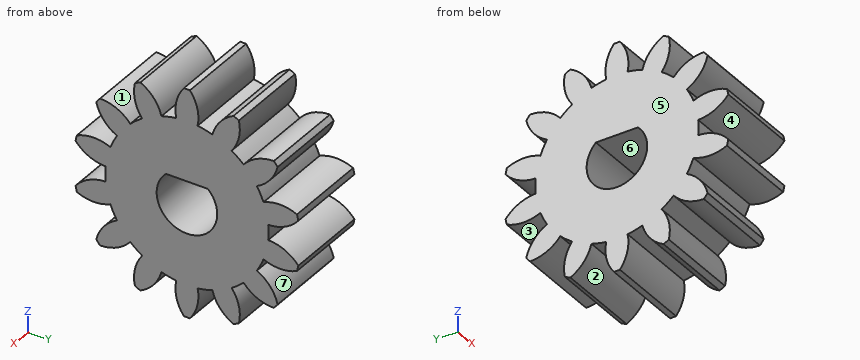
```python
from build123d import *

# Parameters (mm, degrees)
BASPROSKE_W         = 14
BASPROSKE_H         = 12
TOOTHCUT_DEPTH      = 23
TEETHCUTS_COUNT     = 14
TEETHCUTS_ANGLE     = 334.285714286
BORSKE_R            = 3
BORE_DEPTH          = 50.0000508
SKETCH2_R           = 16.086266861
CUT_EXTRUDE1_DEPTH  = 5
SKETCH3_R           = 3.2
CUT_EXTRUDE2_DEPTH  = 20.064015522
BOSS_EXTRUDE1_DEPTH = 9


with BuildPart() as part:
    # BasProSke → Base-Revolve (revolve)
    with BuildSketch(Plane(origin=(0, 0, 0), x_dir=(1, 0, 0), z_dir=(0, 1, 0)), mode=Mode.PRIVATE) as base_revolve_sk:
        with Locations((7, 6)):
            Rectangle(BASPROSKE_W, BASPROSKE_H)
    revolve(base_revolve_sk.sketch.rotate(Axis((-10, 0, 0), (1, 0, 0)), 180), axis=Axis((-10, 0, 0), (1, 0, 0)))

    # TooCutSke → ToothCut (cut, through all)
    with BuildSketch(Plane(origin=(0, 0, 0), x_dir=(0, 0, -1), z_dir=(1, 0, 0))):
        with BuildLine():
            ThreePointArc((0.804845511, 8.586361261), (0, 8.624), (-0.804845511, 8.586361261))
            ThreePointArc((-0.804845511, 8.586361261), (-1.237812142, 10.362618414), (-2.384428228, 11.78663426))
            ThreePointArc((-2.384428228, 11.78663426), (0, 12.0254), (2.384428228, 11.78663426))
            ThreePointArc((2.384428228, 11.78663426), (1.237812142, 10.362618414), (0.804845511, 8.586361261))
        make_face()
    toothcut = extrude(amount=TOOTHCUT_DEPTH, mode=Mode.SUBTRACT)

    # TeethCuts: ToothCut ×14 about axis
    teethcuts_axis = Axis((-10, 0, 0), (1, 0, 0))
    for i in range(1, TEETHCUTS_COUNT):
        add(toothcut.rotate(teethcuts_axis, i * TEETHCUTS_ANGLE / (TEETHCUTS_COUNT - 1)), mode=Mode.SUBTRACT)

    # BorSke → Bore (cut, symmetric)
    with BuildSketch(Plane(origin=(0, 0, 0), x_dir=(0, 0, -1), z_dir=(1, 0, 0))):
        with Locations(Location((0, 0, 0), (0, 0, 180))):
            Circle(BORSKE_R)
    extrude(amount=BORE_DEPTH, both=True, mode=Mode.SUBTRACT)

    # Sketch2 → Cut-Extrude1 (cut)
    with BuildSketch(Plane(origin=(14, 0, 0), x_dir=(0, 0, -1), z_dir=(1, 0, 0))):
        Circle(SKETCH2_R)
    extrude(amount=-CUT_EXTRUDE1_DEPTH, mode=Mode.SUBTRACT)

    # Sketch3 → Cut-Extrude2 (cut, through all)
    with BuildSketch(Plane(origin=(9, 0, 0), x_dir=(0, 0, -1), z_dir=(1, 0, 0))):
        Circle(SKETCH3_R)
    extrude(amount=-CUT_EXTRUDE2_DEPTH, mode=Mode.SUBTRACT)

    # Sketch4 → Boss-Extrude1 (add)
    with BuildSketch(Plane(origin=(9, 0, 0), x_dir=(0, 0, -1), z_dir=(1, 0, 0))):
        with BuildLine():
            Line((-2.3, 2.224859546), (-2.3, -2.224859546))
            ThreePointArc((-2.3, -2.224859546), (-3.2, 0), (-2.3, 2.224859546))
        make_face()
    extrude(amount=-BOSS_EXTRUDE1_DEPTH)


solid = part.part
```
CAD build for the part. Positions are in the model's coordinates, mm. Face numbers are marked on the shaded views. A direction names the side the tool comes from. Coordinates: 2 decimals unless noted, no trailing zeros. Order: outer loops, then holes, each group sorted by start corner. A loop starts at its lowest first (then second) coordinate and runs counter-clockwise, first axis right, second up.
(1) Saw through at D-D, the plane z = 9.5. Write the cut outline in (x, y).
Solution:
outline: (0, -5.58) - (9, -5.58) - (9, -3.27) - (0, -3.27) - close; (0, -1.21) - (9, -1.21) - (9, 1.21) - (0, 1.21) - close; (0, 3.27) - (9, 3.27) - (9, 5.58) - (0, 5.58) - close
(2) Which spindle directions (+Z, -Z, +X, -X, +Y, -Y) get a long thin tool onto all of the face, cutting with end or side? Do the marked faces 1, 2, 3 and 4. Say none if no direction does.
Solution:
face 1: +Z, +X, -X
face 2: -Z, +X, -X
face 3: +X, -X
face 4: +X, -X, -Y
(3) Mould opens along Y. For the marked faces 5, 6 and 7 say: released by +Y, released by -Y, zero draft, split by the parting line, or undercut.
Solution:
face 5: zero draft
face 6: undercut
face 7: released by +Y
(4) Saw through at B-B, the plane y = 0. Write the cut outline in (x, z), and give its area (4 significant figures).
Solution:
outline: (0, -12) - (9, -12) - (9, -3.2) - (0, -3.2) - close; (0, 2.3) - (9, 2.3) - (9, 12) - (0, 12) - close
area: 166.5 mm2
(5) Saw through at A-A, the plane z = 0. Write the cut outline in (x, y), and give its area (3 significant figures).
Solution:
outline: (0, -8.62) - (9, -8.62) - (9, -3.2) - (0, -3.2) - close; (0, 3.2) - (9, 3.2) - (9, 8.62) - (0, 8.62) - close
area: 97.6 mm2
(6) Saw through at C-C, the plane z = -6.75. Write the cut outline in (x, y).
Solution:
outline: (0, -9.43) - (9, -9.43) - (9, -6.52) - (0, -6.52) - close; (0, -5.37) - (9, -5.37) - (9, 5.37) - (0, 5.37) - close; (0, 6.52) - (9, 6.52) - (9, 9.43) - (0, 9.43) - close
(7) Drill centre lines: L1, parallel to Y at x = 6.75, z = 0; L2, parallel to Z at x = 2, y = 0; L3, parallel to Z at x = 5.75, y = -8.5. Where is each one in solid material? Low to high.
Solution:
L1: y = -8.62 to -3.2, 3.2 to 8.62
L2: z = -12 to -3.2, 2.3 to 12
L3: z = -7.67 to -5.27, -3.16 to 3.16, 5.27 to 7.67
(8) Pin check, flat tips, straight feed: pin 1 Ø1.5 at (x, y) = (6, 9) entering from +Z; pin 2 Ø2 at (x, y) = (7, -3.5) entering from +Z; pin 3 Ø5 at (x, y) = (5, -3) entering from -Z. Stop position of each tip, or through.
Solution:
pin 1: stops at z = 7.73
pin 2: stops at z = 10.71
pin 3: stops at z = -11.75
